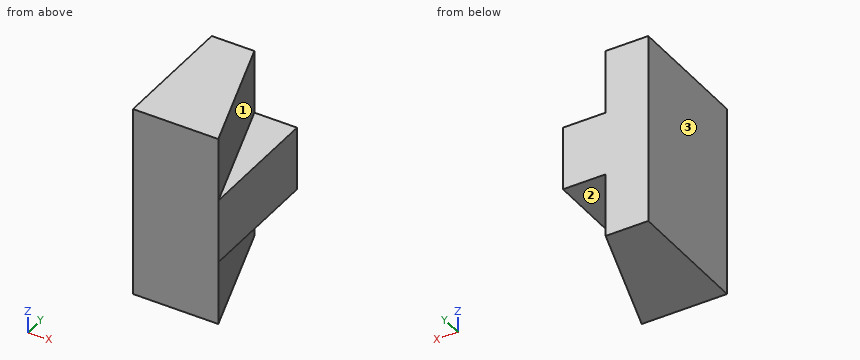
from build123d import *

# Parameters (mm, degrees)
BOSS_EXTRUDE1_DEPTH = 45
BOSS_EXTRUDE2_DEPTH = 15


with BuildPart() as part:
    # Sketch1 → Boss-Extrude1 (new, symmetric)
    with BuildSketch(Plane.XY):
        Polygon((40, 0), (20, 60), (0, 60), (0, 0), align=None)
    extrude(amount=BOSS_EXTRUDE1_DEPTH, both=True)

    # Sketch1_3 → Boss-Extrude2 (add, symmetric)
    with BuildSketch(Plane.XY):
        Polygon((40, 60), (20, 60), (40, 0), align=None)
    extrude(amount=BOSS_EXTRUDE2_DEPTH, both=True)


solid = part.part
Input: part model. Units: mm. Frame: model coordinates. Face numbers are marked on the shaded views. A direction names the side the tool comes from. Give positions to 0.01 mm unless a question says otherwise; leave off trailing zeros. Loops run counter-clockwise (first coordinate to the right, second up) from the corner with the lowest first, then second, coordinate; pieces in that order, holes last. Notation, with made-up numbers: (-13, -21.5) -> (-3, -21.5) arc R30 ccw to (-3, 6.5) -> close; hole circle Ø11 at (13, -35.5). An arc over 180 degrees is marked (long way). Answer as a JSON object with one key per item and string values. Group by question number.
Item 1: Cut plane C-C, the plane z = -31.5. Return the cut outline in (x, y), and give its area (3 significant figures).
Item 2: Reachability of the marked faces 1, 2 and 3 from +Z, -Z, +X, -X, +Y, -Y: full face, straight path, thin tool, end or side. Return the list, or none.
Item 3: Cut plane A-A, the plane x = 34.5. Return the cut outline in (y, z), and give its area (3 significant figures).
Item 4: Cut plane B-B, the plane y = 16.5. Return the cut outline in (x, z).
Item 5: Line query: probe 1 along Z at (x, y) = (38, 46); probe 2 along X at (y, z) = (4.5, 28.5); probe 3 along X at (y, z) = (46, -22). Output: solid intervals per line, ascending.
Checks:
{
 "1": {"outline": "(0, 0) -> (40, 0) -> (20, 60) -> (0, 60) -> close", "area": "1,800 mm²"},
 "2": {"face 1": "+Z, +X, +Y", "face 2": "-Z, +X, +Y", "face 3": "+Z, -Z, -X, +Y, -Y"},
 "3": {"outline": "(0, -45) -> (16.5, -45) -> (16.5, -15) -> (60, -15) -> (60, 15) -> (16.5, 15) -> (16.5, 45) -> (0, 45) -> close", "area": "2,790 mm²"},
 "4": {"outline": "(0, -45) -> (34.5, -45) -> (34.5, -15) -> (40, -15) -> (40, 15) -> (34.5, 15) -> (34.5, 45) -> (0, 45) -> close"},
 "5": {"probe 1": "z = -15 to 15", "probe 2": "x = 0 to 38.5", "probe 3": "x = 0 to 24.67"}
}
